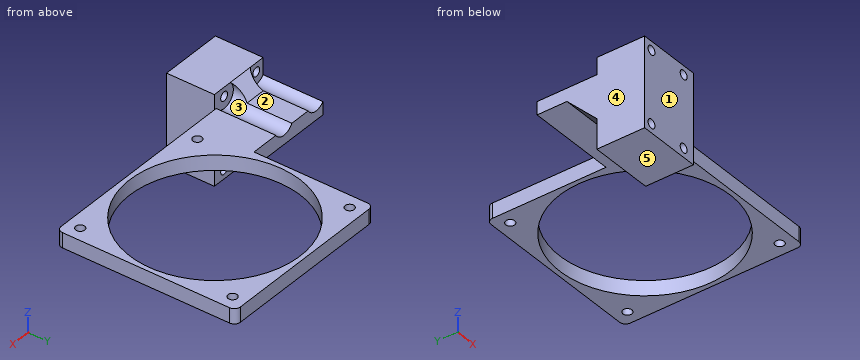
from build123d import *

# Parameters (mm, degrees)
SKETCH_1_W          = 60
SKETCH_1_H          = 60
EXTRUDE_1_DEPTH     = 5
SKETCH_2_R          = 1.5
CUT_EXTRUDE_1_DEPTH = 5
SKETCH_3_R          = 28.5
CUT_EXTRUDE_2_DEPTH = 5
SKETCH_4_W          = 5
SKETCH_4_H          = 20
EXTRUDE_2_DEPTH     = 30
SKETCH_5_W          = 21.25
SKETCH_5_H          = 30
EXTRUDE_3_DEPTH     = 16
SKETCH_6_R          = 1.5
CUT_EXTRUDE_3_DEPTH = 30
SKETCH_7_R          = 4
CUT_EXTRUDE_4_DEPTH = 30
CHAMFER_1_SIZE      = 10
CHAMFER_2_SIZE      = 5
FILLET_1_R          = 2


with BuildPart() as part:
    # 草图1 → 凸台-拉伸1 (new body)
    with BuildSketch(Plane.XY):
        with Locations((-30, 30)):
            Rectangle(SKETCH_1_W, SKETCH_1_H)
    extrude(amount=EXTRUDE_1_DEPTH)

    # 草图2 → 切除-拉伸1 (cut)
    with BuildSketch(Plane(origin=(0, 0, 0), x_dir=(-1, 0, 0), z_dir=(0, 0, -1))):
        with Locations((4.5, 55.5)):
            Circle(SKETCH_2_R)
        with Locations((55.5, 55.5)):
            Circle(SKETCH_2_R)
        with Locations((4.5, 4.5)):
            Circle(SKETCH_2_R)
        with Locations((55.5, 4.5)):
            Circle(SKETCH_2_R)
    extrude(amount=-CUT_EXTRUDE_1_DEPTH, mode=Mode.SUBTRACT)

    # 草图3 → 切除-拉伸2 (cut)
    with BuildSketch(Plane(origin=(0, 0, 0), x_dir=(-1, 0, 0), z_dir=(0, 0, -1))):
        with Locations((30, 30)):
            Circle(SKETCH_3_R)
    extrude(amount=-CUT_EXTRUDE_2_DEPTH, mode=Mode.SUBTRACT)

    # 草图4 → 凸台-拉伸2 (add)
    with BuildSketch(Plane.ZY.offset(60)):
        with Locations((2.5, 10)):
            Rectangle(SKETCH_4_W, SKETCH_4_H)
    extrude(amount=EXTRUDE_2_DEPTH)

    # 草图5 → 凸台-拉伸3 (add)
    with BuildSketch(Plane.XZ):
        with Locations((-79.375, -5)):
            Rectangle(SKETCH_5_W, SKETCH_5_H)
    extrude(amount=EXTRUDE_3_DEPTH)

    # 草图6 → 切除-拉伸3 (cut)
    with BuildSketch(Plane.XZ.offset(16)):
        with Locations(Location((-87, 7, 0), (0, 0, 270))):
            Circle(SKETCH_6_R)
        with Locations(Location((-73, 7, 0), (0, 0, 270))):
            Circle(SKETCH_6_R)
        with Locations(Location((-87, -17, 0), (0, 0, 270))):
            Circle(SKETCH_6_R)
        with Locations(Location((-73, -17, 0), (0, 0, 270))):
            Circle(SKETCH_6_R)
    extrude(amount=-CUT_EXTRUDE_3_DEPTH, mode=Mode.SUBTRACT)

    # 草图7 → 切除-拉伸4 (cut)
    with BuildSketch(Plane(origin=(0, 0, 0), x_dir=(1, 0, 0), z_dir=(0, 1, 0))):
        with Locations((-87, -7)):
            Circle(SKETCH_7_R)
        with Locations((-73, -7)):
            Circle(SKETCH_7_R)
    extrude(amount=CUT_EXTRUDE_4_DEPTH, mode=Mode.SUBTRACT)

    # 倒角1
    chamfer_1_edges = [part.edges().sort_by_distance(p)[0] for p in [
        (-79.375, 0, 0),
    ]]
    chamfer(chamfer_1_edges, length=CHAMFER_1_SIZE)

    # 倒角2
    chamfer_2_edges = [part.edges().sort_by_distance(p)[0] for p in [
        (-80, 0, 5),
    ]]
    chamfer(chamfer_2_edges, length=CHAMFER_2_SIZE - 0.0001)  # a hair under: the kernel refuses the full size

    # 圆角1
    fillet_1_edges = [part.edges().sort_by_distance(p)[0] for p in [
        (0, 0, 2.5),
        (-60, 60, 2.5),
        (0, 60, 2.5),
    ]]
    fillet(fillet_1_edges, radius=FILLET_1_R)


solid = part.part
For this review, take the finished solid that the model builds, in its own axes (mm). Face numbers are marked on the shaded views. A direction names the side the tool comes from. Round coordinates to 2 decimals unless told otherwise and drop trailing zeros. Loops run counter-clockwise (first coordinate to the right, second up) from the corner with the lowest first, then second, coordinate; pieces in that order, holes last. Notation, with made-up numbers: (63.5, 81) - (101.5, 81) arc R24 cw to (101.5, 119) - close; hole circle Ø11 at (30.25, 66.25). An arc over 180 degrees is marked (long way). Use one line per item in the form item = value.
Item 1: Mouldability with a two-part tool opening along X and no side actions: class the marked faces 3, 4 and 5 as +X half, -X half, draft (parallel to the pull), parting line (faces both ways), or undercut.
Answers:
face_3 = undercut
face_4 = -X half
face_5 = draft
Item 2: Consider section A-A on y = 30. Write out the cut boundary in (x, z), then the cut area to 3 significant figures.
Answers:
outline = (-60, 0) - (-58.5, 0) - (-58.5, 5) - (-60, 5) - close; (-1.5, 0) - (0, 0) - (0, 5) - (-1.5, 5) - close
area = 15.0 mm^2
Item 3: Clearance check with flat-ended pins moving along their axes: P1, Ø1.5, axis at x = -78, z = 3.5, coming from the +Y side; P2, Ø5, axis at x = -4.5, y = 55.5, coming from the +Z side; P3, Ø1.8, axis at x = -87, z = -17, coming from the +Y side; P4, Ø2, axis at x = -83, z = 6.5, coming from the +Y side. State where each tip first meets the part, or that it passes through.
Answers:
P1 = 20
P2 = 5
P3 = through
P4 = 4.5
Item 4: For line 1 (Z direction, x = -73, y = -3); line 2 (X direction, y = -12, z = 7); line 3 (Y direction, x = -4.5, z = 2.75), list the stretches that pass through material, from the lowest coordinate up.
Answers:
line_1 = -20 to -18.5, -15.5 to 5.5, 8.5 to 10
line_2 = -90 to -88.5, -85.5 to -74.5, -71.5 to -68.75
line_3 = 0 to 3, 6 to 17.27, 42.73 to 54, 57 to 60
Item 5: Consider section B-B on x = -73. Write out the cut boundary in (y, z), then the cut area to 3 significant figures.
Answers:
outline = (-16, -20) - (0, -20) - (0, -18.5) - (-16, -18.5) - close; (-16, -15.5) - (0, -15.5) - (0, -10) - (10, 0) - (20, 0) - (20, 3) - (0, 3) - (0, 5.5) - (-16, 5.5) - close; (-16, 8.5) - (0, 8.5) - (0, 10) - (-16, 10) - close
area = 494 mm^2
Item 6: Consider section C-C on z = 6.75. Write out the cut boundary in (x, y).
Answers:
outline = (-90, -16) - (-88.48, -16) - (-88.48, 0) - (-90, 0) - close; (-85.52, -16) - (-74.48, -16) - (-74.48, 0) - (-76.99, 0) - (-76.99, 3.25) - (-83.01, 3.25) - (-83.01, 0) - (-85.52, 0) - close; (-71.52, -16) - (-68.75, -16) - (-68.75, 0) - (-71.52, 0) - close
Item 7: Tool access review of the marked faces 1 and 2: name each direction out of +Z, -Z, +X, -X, +Y, -Y from which nothing blocks a thin tool from reaching the whole face with its end or side.
Answers:
face_1 = +Z, -Z, +X, -X, -Y
face_2 = +Z, +X, -X, +Y
Item 8: Consider section D-D on x = -9. Write out the cut boundary in (y, z).
Answers:
outline = (0, 0) - (10.73, 0) - (10.73, 5) - (0, 5) - close; (49.27, 0) - (60, 0) - (60, 5) - (49.27, 5) - close
